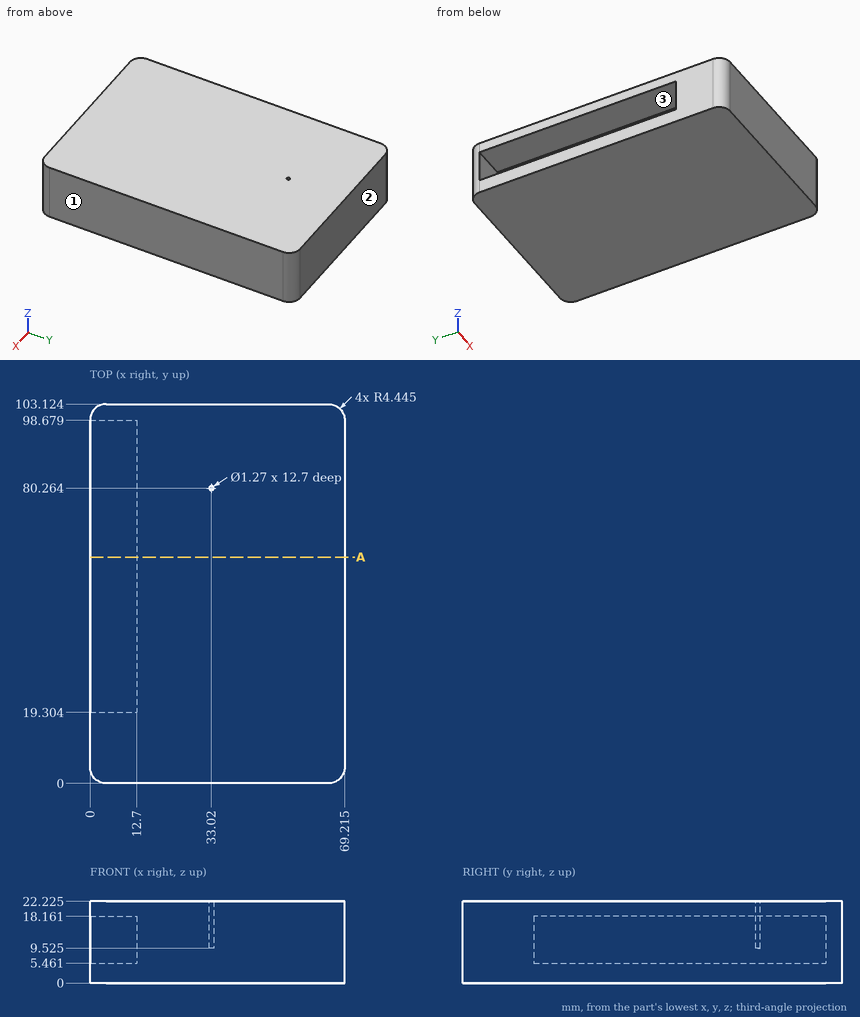
Geometry check sheet. Reference: drawing and pictorial views, mm from the part's lowest x, y, z. Give positions to 0.01 mm unless a question says otherwise; leave off trailing zeros. Order: outer loops, then holes, each group sorted by start corner. A loop starts at its lowest first (then second) coordinate and runs counter-clockwise, first axis right, second up. Notation, with made-up numbers: M -2.5,86 L 36.5,86 A19 ccw 36.5,111 Z; hole C -8,9 d1. An arc over 180 degrees is marked long. Answer in a Markdown table with one row per item. Add a question column.
Item 1: Mould release check, pull along Y, two halves, no side actions. Record for the marked faces 1, 2 and 3: released by +Y, released by -Y, zero draft, split by the parting line, or undercut.
Item 2: Scan lines: probe 1 along Z at (x, y) = (10.5, 55) (3 decimals); probe 2 along Y at (x, z) = (33, 19); probe 3 along X at (y, z) = (94, 6.25) (3 decimals). Record each from-to range of solid material in increasing order. Write a range as from..to.
Item 3: Section check A-A, the plane y = 61.5. Enter the section's corners in (x, z) (3 decimals).
Filled sheet:
| question | item | result |
|---|---|---|
| 1 | face 1 | zero draft |
| 1 | face 2 | released by +Y |
| 1 | face 3 | undercut |
| 2 | probe 1 | z = 0..5.461, 18.161..22.225 |
| 2 | probe 2 | y = 0..79.63, 80.9..103.12 |
| 2 | probe 3 | x = 12.7..69.215 |
| 3 | outline | M 0,0 L 69.215,0 L 69.215,22.225 L 0,22.225 L 0,18.161 L 12.7,18.161 L 12.7,5.461 L 0,5.461 Z |
